Source: CAD feature listing. Evaluate the final solid. Frame: model axes, mm. Face numbers are marked on the shaded views. A direction names the side the tool comes from. Give positions to 0.01 mm unless a question says otherwise; leave off trailing zeros. Write each loop counter-clockwise with the first axis right and the second up, starting at its lowest first coordinate (ties: lowest second). Pieces come first, ordered by that corner, then holes. Notation, with made-up numbers: (26, 49.5) -> (71, 49.5) arc R17 ccw to (71, 75.5) -> close; hole circle Ø2 at (20.25, 0). An arc over 180 degrees is marked (long way). Answer as a JSON object with one key per item and string values. Group by question number.
Item 1: Pull-direction query (X, two-part tool) for the marked faces 4, 5, 6 and 7; classes: pulls with the +X half, pulls with the -X half, needs draft (parallel to the pull), parting line crosses it, or undercut.
Item 2: Section query D-D on y = -3.5. Return the cut outline in (x, z).
Item 3: Access query for the marked faces 1, 2 and 3. Directions: +Z, -Z, +X, -X, +Y, -Y. A direction counts if a zero-diameter tool reaches every point of the face in a straight line with its end or side. Return the directions, or none.
Item 4: First-contact query: pin 1 Ø6.5 at (x, z) = (-2.5, 7.5) entering from -Y; pin 2 Ø1.6 at (x, z) = (0.5, 0.5) entering from -Y; pin 3 Ø4 at (x, y) = (8, -2.5) entering from -Z; pin 4 Ø1 at (y, z) = (-2.5, 14) entering from +X. Flat tips, straight axial feed; report the tip coordinate or a pass-through.
Item 5: Section query B-B on x = 6. Return the cut outline in (y, z).
Item 6: Section query C-C on z = 0. Return the cut outline in (x, y), plus the area to 3 significant figures.
Item 7: Ray query, probe 1 along Y at (x, z) = (-0.5, 8.5); probe 2 along Z at (x, y) = (1.5, 1.5); probe 3 along Z at (x, y) = (0.25, -1.25). Return the intervals inside material, ascending. Write a range as from..to.
Item 8: Section query A-A on x = 0. Return the cut outline in (y, z) (3 decimals).
from build123d import *

# Parameters (mm, degrees)
CROQUIS1_W                          = 20
CROQUIS1_H                          = 3.5
SALIENTE_EXTRUIR1_DEPTH             = 4
CROQUIS2_R                          = 1
SALIENTE_EXTRUIR2_DEPTH             = 2
CROQUIS3_W                          = 20
CROQUIS3_H                          = 2
SALIENTE_EXTRUIR3_DEPTH             = 8
CROQUIS4_W                          = 20
CROQUIS4_H                          = 1.732050807
SALIENTE_EXTRUIR4_DEPTH             = 12
SALIENTE_EXTRUIR4_DIRECTION_2_REACH = 17.06
CROQUIS5_R                          = 1.75
CORTAR_EXTRUIR1_DEPTH               = 23.571551689


with BuildPart() as part:
    # Croquis1 → Saliente-Extruir1 (new body)
    with BuildSketch(Plane(origin=(0, 0, 0), x_dir=(1, 0, 0), z_dir=(0, 1, 0))):
        Rectangle(CROQUIS1_W, CROQUIS1_H)
    extrude(amount=SALIENTE_EXTRUIR1_DEPTH)

    # Croquis2 → Saliente-Extruir2 (add)
    with BuildSketch(Plane.XZ):
        with Locations(Location((0, 0, 0), (0, 0, 270))):
            Circle(CROQUIS2_R)
        with Locations(Location((-6, 0, 0), (0, 0, 90))):
            Circle(CROQUIS2_R)
        with Locations(Location((6, 0, 0), (0, 0, 90))):
            Circle(CROQUIS2_R)
    extrude(amount=SALIENTE_EXTRUIR2_DEPTH)

    # Croquis3 → Saliente-Extruir3 (add)
    with BuildSketch(Plane.XY.offset(1.75)):
        with Locations((0, 3)):
            Rectangle(CROQUIS3_W, CROQUIS3_H)
    extrude(amount=SALIENTE_EXTRUIR3_DEPTH)

    # Croquis4 → Saliente-Extruir4 (add)
    with BuildSketch(Plane(origin=(0, -3.721873843, 6.446474596), x_dir=(1, 0, 0), z_dir=(0, -0.500000000000001, 0.866025403784438))):
        with Locations((0, 7.473076212)):
            Rectangle(CROQUIS4_W, CROQUIS4_H)
    extrude(amount=SALIENTE_EXTRUIR4_DEPTH)

    # Croquis4 → Saliente-Extruir4 direction 2 (add, up to next)
    with BuildSketch(Plane(origin=(0, -3.721873843, 6.446474596), x_dir=(1, 0, 0), z_dir=(0, -0.500000000000001, 0.866025403784438)), mode=Mode.PRIVATE) as saliente_extruir4_direction_2_sk1:
        with Locations((0, 7.473076212)):
            Rectangle(CROQUIS4_W, CROQUIS4_H)
    saliente_extruir4_direction_2_tool1 = extrude(saliente_extruir4_direction_2_sk1.sketch, amount=-SALIENTE_EXTRUIR4_DIRECTION_2_REACH, mode=Mode.PRIVATE) - part.part
    add(saliente_extruir4_direction_2_tool1.solids().sort_by_distance((0, 2.75, 10.183013))[0])

    # Croquis5 → Cortar-Extruir1 (cut, through all)
    with BuildSketch(Plane(origin=(0, 7.221873843, 4.169550808), x_dir=(1, 0, 0), z_dir=(0, 0.8660254037844382, 0.500000000000001))):
        with Locations(Location((0, -12.943747687, 0), (0, 0, 270))):
            Circle(CROQUIS5_R)
    extrude(amount=-CORTAR_EXTRUIR1_DEPTH, mode=Mode.SUBTRACT)


solid = part.part
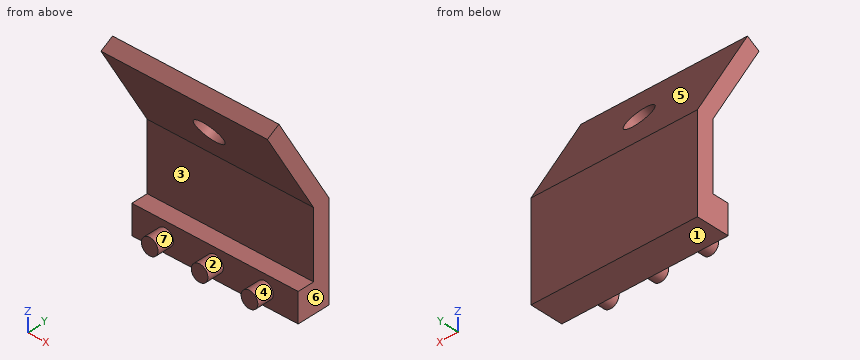
Worked answers:
{
 "1": {"face 4": "undercut", "face 5": "needs draft", "face 6": "pulls with the +X half", "face 7": "undercut"},
 "2": {"outline": "(-10, 19.28) -> (10, 19.28) -> (10, 20.43) -> (-10, 20.43) -> close"},
 "3": {"face 1": "-Z, +X, -X, +Y, -Y", "face 2": "-Y", "face 3": "+X, -X, -Y"},
 "4": {"pin 1": "y = 1.42", "pin 2": "y = -2", "pin 3": "z = -1", "pin 4": "through"},
 "5": {"outline": "(-4, 20.14) -> (2, 9.75) -> (2, 1.75) -> (0, 1.75) -> (0, 1) -> (-2, 1) -> (-2, -1) -> (0, -1) -> (0, -1.75) -> (4, -1.75) -> (4, 9.75) -> (-2.5, 21.01) -> close"},
 "6": {"outline": "(-10, 0) -> (-7, 0) -> (-7, -2) -> (-5, -2) -> (-5, 0) -> (-1, 0) -> (-1, -2) -> (1, -2) -> (1, 0) -> (5, 0) -> (5, -2) -> (7, -2) -> (7, 0) -> (10, 0) -> (10, 4) -> (-10, 4) -> close", "area": "92.0 mm^2"},
 "7": {"probe 1": "2..4", "probe 2": "-1.75..1.75, 10.62..14.08", "probe 3": "-0.97..0.97, 16.22..18.84"},
 "8": {"outline": "(-4, 20.142) -> (-1.625, 16.029) -> (-0.125, 16.895) -> (-2.5, 21.008) -> close; (-2, -1) -> (0, -1) -> (0, -1.75) -> (4, -1.75) -> (4, 9.75) -> (1.625, 13.864) -> (0.125, 12.998) -> (2, 9.75) -> (2, 1.75) -> (0, 1.75) -> (0, 1) -> (-2, 1) -> close"}
}
